Solid Edge part; units mm, degrees
sketch "Sketch1" plane through (0, 0, 0) normal (0, 0, 1) x (1, 0, 0)
  circle A0 centre (0, 0) radius 1.25
extrude "Protrusion1" add sketch "Sketch1" along normal blind 60
sketch "Sketch2" plane through (0, 0, 29.23) normal (0, 0, 1) x (1, 0, 0)
  circle A0 centre (0, 0) radius 1.425
extrude "ExtrudedProtrusion_2" add sketch "Sketch2" against normal blind 5.33
Here's how the part is built. I have some questions about the finished solid (model axes, mm). A direction names the side the tool comes from. Coordinates: 2 decimals unless noted, no trailing zeros. Order: outer loops, then holes, each group sorted by start corner. A loop starts at its lowest first (then second) coordinate and runs counter-clockwise, first axis right, second up. Notation, with made-up numbers: M 36,-1 L 67,-1 A18 ccw 67,9 Z; hole C 58.5,30.5 d2. An arc over 180 degrees is marked long. Answer as a JSON object with one key per item and string values. Group by question number.
(1) Which directions (+Z, -Z, +X, -X, +Y, -Y) give clear straight access to the entire face, cutting with the end or side of a thin tool? Please do faces 1 (the face through (-0.27, 1.22, 11.78)), 2 (the face through (-0.27, 1.22, 44.4)), 3 (the face through (0, 0, 0)).
(2) Suppose I cut it at A-A, the plane y = 0. Please give me the cut outline in (x, z) (3 decimals).
(3) Suppose I cut it at C-C, the plane z = 30.5. Please give me the cut outline in (x, y), then the cut area to 3 significant figures.
(4) For pin 1 (1.5 mm diameter, centred on y = 1, z = 22, fed in from -X); pin 2 (1.5 mm diameter, centred on y = -0.5, z = 29.5, fed in from -X) (3 decimals), each with a flat end and sliding along its axis, tell me the tip position at first contact or that it passes through.
(5) I need wall thicknesses on probe 1 along X at (y, z) = (-0.1, 14); probe 2 along Y at (x, z) = (-1, 12.5). Which ranges of each line are inside material? Lowest first, please.
Values found:
{
 "1": {"face 1": "-Z", "face 2": "+Z", "face 3": "-Z, +X, -X, +Y, -Y"},
 "2": {"outline": "M -1.425,23.9 L -1.25,23.9 L -1.25,0 L 1.25,0 L 1.25,23.9 L 1.425,23.9 L 1.425,29.23 L 1.25,29.23 L 1.25,60 L -1.25,60 L -1.25,29.23 L -1.425,29.23 Z"},
 "3": {"outline": "C 0,0 d2.5", "area": "4.91 mm^2"},
 "4": {"pin 1": "stops at x = -1.22", "pin 2": "stops at x = -1.425"},
 "5": {"probe 1": "x = -1.25 to 1.25", "probe 2": "y = -0.75 to 0.75"}
}
